CAD build for the part. Positions are in the model's coordinates, mm. A direction names the side the tool comes from. Round coordinates to 2 decimals unless told otherwise and drop trailing zeros. Order: outer loops, then holes, each group sorted by start corner. A loop starts at its lowest first (then second) coordinate and runs counter-clockwise, first axis right, second up. Notation, with made-up numbers: M 64,65 L 122,65 A22 ccw 122,89 Z; hole C 28,75 d1. An arc over 180 degrees is marked long. Answer as a JSON object with one key per item and string values. Group by question number.
```python
from build123d import *

# Parameters (mm, degrees)
F0_W     = 17.4
F0_H     = 6.2
F1_DEPTH = 1
F0_W_2   = 19.4
F0_H_2   = 8.2
F2_DEPTH = 9
F3_W     = 4
F3_H     = 7
F4_DEPTH = 2
F5_W     = 0.6
F5_H     = 0.6
F6_DEPTH = 25


with BuildPart() as f1:
    # F0 (on Top) → F1 (new body)
    with BuildSketch(Plane.XY):
        with Locations((1.278801, 13.346958)):
            Rectangle(F0_W, F0_H)
    extrude(amount=F1_DEPTH)

    # F0 (on Top) → F2 (join)
    with BuildSketch(Plane.XY):
        with Locations((1.278801, 13.346958)):
            Rectangle(F0_W_2, F0_H_2)
        with Locations((1.278801, 13.346958)):
            Rectangle(F0_W, F0_H, mode=Mode.SUBTRACT)
    extrude(amount=F2_DEPTH)

    # F3 (on face) → F4 (cut)
    with BuildSketch(Plane.XZ.offset(-9.246958)):
        with Locations((1.278801, 5.5)):
            Rectangle(F3_W, F3_H)
    extrude(amount=-F4_DEPTH, mode=Mode.SUBTRACT)

    # F5 (on face) → F6 (cut)
    with BuildSketch(Plane.XY.offset(1)):
        with Locations((-3.801199, 11.958958)):
            Rectangle(F5_W, F5_H)
        with Locations((-3.801199, 14.498958)):
            Rectangle(F5_W, F5_H)
        with Locations((-1.261199, 14.498958)):
            Rectangle(F5_W, F5_H)
        with Locations((-1.261199, 11.958958)):
            Rectangle(F5_W, F5_H)
        with Locations((1.278801, 11.958958)):
            Rectangle(F5_W, F5_H)
        with Locations((1.278801, 14.498958)):
            Rectangle(F5_W, F5_H)
        with Locations((3.818801, 11.958958)):
            Rectangle(F5_W, F5_H)
        with Locations((3.818801, 14.498958)):
            Rectangle(F5_W, F5_H)
        with Locations((6.358801, 14.498958)):
            Rectangle(F5_W, F5_H)
        with Locations((6.358801, 11.958958)):
            Rectangle(F5_W, F5_H)
    extrude(amount=-F6_DEPTH, mode=Mode.SUBTRACT)


solid = f1.part
```
Item 1: Cut at C-C, the plane y = 10. Give the cut face in (x, z).
Item 2: Cut at D-D, the plane x = -5. Give the cut face in (y, z).
Item 3: Cut at A-A, the plane z = 1.25. Give the cut face in (x, y), and give its area (3 significant figures).
Item 4: Drill centre lines: line 1 (Y direction, x = -3.75, z = 0.75); line 2 (X direction, y = 13.5, z = 3); line 3 (Y direction, x = -0.25, z = 1.75). Where is each one in solid material? Low to high. Write a range as [from, to].
Item 5: 3-axis set-ups, long thin cutter, end or side, ignore diameter. For faces 1 (the face through (-8.421, 13, 4)), 2 (the face through (9.979, 13, 5)), 3 (the face through (1, 10, 2)): which of +Z, -Z, +X, -X, +Y, -Y reach the whole face in a straight line?
Item 6: Cut at B-B, the plane y = 12. Give the cut face in (x, z).
Item 7: Two-plate mould, pull along X, no slides. Class faces 4 (the face through (1, 17, 9)), 5 (the face through (10.979, 13, 4)), 6 (the face through (3.279, 10, 5)), 7 (the face through (-0.721, 10, 5)): +X half, -X half, draft (parallel to the pull), parting line (faces both ways), or undercut.
Response values:
{
 "1": {"outline": "M -8.42,0 L 10.98,0 L 10.98,9 L 3.28,9 L 3.28,2 L -0.72,2 L -0.72,9 L -8.42,9 Z"},
 "2": {"outline": "M 9.25,0 L 17.45,0 L 17.45,9 L 16.45,9 L 16.45,1 L 10.25,1 L 10.25,9 L 9.25,9 Z"},
 "3": {"outline": "M -8.42,9.25 L 10.98,9.25 L 10.98,17.45 L -8.42,17.45 Z; hole M -7.42,10.25 L 9.98,10.25 L 9.98,16.45 L -7.42,16.45 Z", "area": "51.2 mm^2"},
 "4": {"line 1": "[9.25, 11.66], [12.26, 14.2], [14.8, 17.45]", "line 2": "[-8.42, -7.42], [9.98, 10.98]", "line 3": "[9.25, 10.25], [16.45, 17.45]"},
 "5": {"face 1": "+Z, -Z, -X, +Y, -Y", "face 2": "+Z", "face 3": "+Z, -Y"},
 "6": {"outline": "M -8.42,0 L -4.1,0 L -4.1,1 L -7.42,1 L -7.42,9 L -8.42,9 Z; M -3.5,0 L -1.56,0 L -1.56,1 L -3.5,1 Z; M -0.96,0 L 0.98,0 L 0.98,1 L -0.96,1 Z; M 1.58,0 L 3.52,0 L 3.52,1 L 1.58,1 Z; M 4.12,0 L 6.06,0 L 6.06,1 L 4.12,1 Z; M 6.66,0 L 10.98,0 L 10.98,9 L 9.98,9 L 9.98,1 L 6.66,1 Z"},
 "7": {"face 4": "draft", "face 5": "+X half", "face 6": "undercut", "face 7": "undercut"}
}
